from build123d import *

# Parameters (mm, degrees)
F0_W     = 15.0114
F0_H     = 17.4625
F0_W_2   = 7.2136
F0_H_2   = 10.287
F2_R     = 1.5875
F3_SIZE  = 0.79375
F4_SIZE2 = 6.35
F4_SIZE  = 1.5748


with BuildPart() as f1:
    # F0 (on Right) → F1 (revolve)
    with BuildSketch(Plane.YZ):
        with Locations((14.7193, 16.66875)):
            Rectangle(F0_W, F0_H)
        with Locations((3.6068, 16.66875)):
            Rectangle(F0_W_2, F0_H)
        with Locations((3.6068, 30.5435)):
            Rectangle(F0_W_2, F0_H_2)
    revolve(axis=Axis((0, 11.1125, 0), (0, 1, 0)))

    # F2
    f2_edges = [f1.edges().sort_by_distance(p)[0] for p in [
        (0, 7.2136, -25.4),
    ]]
    fillet(f2_edges, radius=F2_R)

    # F3
    f3_edges = [f1.edges().sort_by_distance(p)[0] for p in [
        (0, 22.225, -25.4),
    ]]
    chamfer(f3_edges, length=F3_SIZE)

    # F4
    f4_edges = [f1.edges().sort_by_distance(p)[0] for p in [
        (0, 7.2136, -35.687),
        (0, 0, -35.687),
        (0, 3.6068, 35.687),
    ]]
    f4_side = f1.faces().sort_by_distance((0, 3.6068, -35.687))[0]
    chamfer(f4_edges, length=F4_SIZE, length2=F4_SIZE2, reference=f4_side)


solid = f1.part
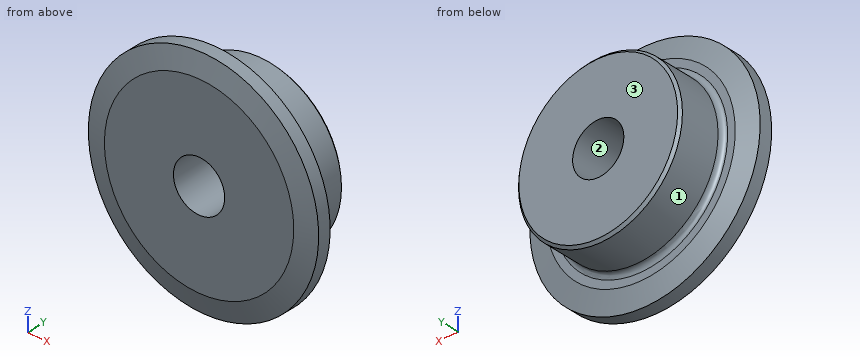
Part model, mm, in its own coordinate system. Face numbers are marked on the shaded views. Give positions to 0.01 mm unless a question says otherwise; leave off trailing zeros. Loops run counter-clockwise (first coordinate to the right, second up) from the corner with the lowest first, then second, coordinate; pieces in that order, holes last. Notation, with made-up numbers: M 49.25,-17.75 L 72.25,-17.75 A12 ccw 72.25,5.25 Z; hole C 87.25,-31 d5. An arc over 180 degrees is marked long. Put each result on its own line as item: value. Start each with the question number.
1) Saw through at A-A (x = 0). List the corners of the cut face in (y, z) (1 decimal).
2) Probe probe 1 along X at (y, z) = (5.25, 0); probe 2 along X at (y, z) = (14.25, 0); probe 3 along Z at (x, y) = (-3.5, 9.75). List the from-to ranges inside material, lowest first.
3) Saw through at B-B (z = 0). List the corners of the cut face in (x, y) (1 decimal), then the cut area to 3 significant figures.
4) Saw through at C-C (y = 3). List the corners of the cut face in (x, z) (1 decimal), then the cut area to 3 significant figures.
5) Pull direction Z, two halves, no side cores. Call the marked faces 1, 2 and 3: +Z half, -Z half, draft (parallel to the pull), parting line (faces both ways), or undercut.
6) Flat gauge pins, fed straight in: pin 1 (1.5 mm diameter, centred on x = 13, z = -28.5, fed in from +Y); pin 2 (6 mm diameter, centred on x = -1, y = 18.5, fed in from -Z); pin 3 (3 mm diameter, centred on y = 12.5, z = -13, fed in from -X). Where does each tip first touch, or does it go through?
Numbers:
1. outline: M 0,-29.3 L 1.6,-35.7 L 5.6,-35.7 L 7.2,-29.3 L 7.2,-27 A1.6 cw 8.8,-25.4 L 21.4,-25.4 L 22.2,-24.6 L 22.2,-7.9 L 0,-7.9 Z; M 0,7.9 L 22.2,7.9 L 22.2,24.6 L 21.4,25.4 L 8.8,25.4 A1.6 cw 7.2,27 L 7.2,29.3 L 5.6,35.7 L 1.6,35.7 L 0,29.3 Z
2. probe 1: -35.69 to -7.94, 7.94 to 35.69
2. probe 2: -25.4 to -7.94, 7.94 to 25.4
2. probe 3: -25.16 to -7.12, 7.12 to 25.16
3. outline: M -35.7,1.6 L -29.3,0 L -7.9,0 L -7.9,22.2 L -24.6,22.2 L -25.4,21.4 L -25.4,8.8 A1.6 cw -27,7.2 L -29.3,7.2 L -35.7,5.6 Z; M 7.9,0 L 29.3,0 L 35.7,1.6 L 35.7,5.6 L 29.3,7.2 L 27,7.2 A1.6 cw 25.4,8.8 L 25.4,21.4 L 24.6,22.2 L 7.9,22.2 Z
3. area: 905 mm^2
4. outline: C 0,0 d71.4; hole C 0,0 d15.9
4. area: 3,800 mm^2
5. face 1: parting line
5. face 2: undercut
5. face 3: draft
6. pin 1: y = 6.91
6. pin 2: z = -25.4
6. pin 3: x = -22.65
